from build123d import *

# Parameters (mm, degrees)
SKETCH1_R           = 2.1
BOSS_EXTRUDE1_DEPTH = 3.175
FILLET2_R           = 1
FILLET3_R           = 1


with BuildPart() as part:
    # Sketch1 → Boss-Extrude1 (new body)
    with BuildSketch(Plane.XY):
        with BuildLine():
            Line((7.553744451, 70.714270531), (-1.524, 70.714270531))
            Line((-1.524, 70.714270531), (-1.524, 132.971298819))
            Line((-1.524, 132.971298819), (-13.246972093, 161.314442451))
            Line((-13.246972093, 161.314442451), (-11.976972093, 161.314442451))
            ThreePointArc((-11.976972093, 161.314442451), (0.849692503, 157.261830841), (10.122503099, 167.006674049))
            Line((10.122503099, 167.006674049), (11.392503099, 167.006674049))
            Line((11.392503099, 167.006674049), (10.2026, 132.971298819))
            Line((10.2026, 132.971298819), (10.2026, 70.714270531))
            Line((10.2026, 70.714270531), (7.553744451, 70.714270531))
        make_face()
        with Locations((4.2926, 126.820276743)):
            Circle(SKETCH1_R, mode=Mode.SUBTRACT)
        with Locations((4.2926, 80.951718801)):
            Circle(SKETCH1_R, mode=Mode.SUBTRACT)
    extrude(amount=BOSS_EXTRUDE1_DEPTH)

    # Fillet2
    fillet2_edges = [part.edges().sort_by_distance(p)[0] for p in [
        (-11.976972093, 161.314442451, 1.5875),
        (10.122503099, 167.006674049, 1.5875),
        (10.2026, 70.714270531, 1.5875),
        (-1.524, 70.714270531, 1.5875),
        (-1.524, 132.971298819, 1.5875),
    ]]
    fillet(fillet2_edges, radius=FILLET2_R)

    # Fillet3
    # the kernel refuses this fillet: 1 mm, written as the material it takes off along each edge
    with BuildSketch(Plane(origin=(-13.246972093, 161.314442451, -3.208100544), x_dir=(1, 0, 0), z_dir=(0, 0, 1))) as fillet3_piece_1:
        with BuildLine():
            CenterArc((1.414539547, -0.803606449), FILLET3_R, 126.524113779, 75.946301344)
            Line((0.490462538, -1.185812782), (0.471980998, -1.193456909))
            Line((0.471980998, -1.193456909), (-0.01848154, -0.007644127))
            Line((-0.01848154, -0.007644127), (0, 0.02))
            ThreePointArc((0, 0.02), (0.409689249, 0.02), (0.807475277, 0.016072129))
            Line((0.807475277, 0.016072129), (0.819378498, 0))
        make_face()
    extrude(amount=9.591201087, mode=Mode.SUBTRACT)
    with BuildSketch(Plane(origin=(11.392503099, 167.006674049, -2.176149378), x_dir=(-1, 0, 0), z_dir=(0, 0, 1))) as fillet3_piece_2:
        with BuildLine():
            CenterArc((1.029802799, 0.834988847), FILLET3_R, 177.997710642, 58.616966228)
            Line((0.030413367, 0.869928276), (0.010425578, 0.870627065))
            Line((0.010425578, 0.870627065), (-0.019987789, 0.000698789))
            Line((-0.019987789, 0.000698789), (0, -0.02))
            ThreePointArc((0, -0.02), (0.239767965, -0.02), (0.468530594, -0.016699777))
            Line((0.468530594, -0.016699777), (0.479535931, 0))
        make_face()
    extrude(amount=7.527298756, mode=Mode.SUBTRACT)


solid = part.part
The listing builds one solid part. Answer for the finished solid, in the listing's coordinates (mm). A direction names the side the tool comes from. Round coordinates to 2 decimals unless told otherwise and drop trailing zeros. Write each loop counter-clockwise with the first axis right and the second up, starting at its lowest first coordinate (ties: lowest second). Pieces come first, ordered by that corner, then holes. Notation, with made-up numbers: M -32.5,31 L -17.5,31 A20 ccw -17.5,39 Z; hole C 86.25,6.5 d8. An arc over 180 degrees is marked long. Write each question's results on one line, items separated by ' | '. Start each with the question number.
(1) The part is cut by section D-D, the plane y = 107.5. Write down the section's boundary in (x, z) (3 decimals).
(2) The part is cut by section B-B, the plane z = 1.9. Write down the section's boundary in (x, y), and give its area (3 significant figures).
(3) The part is cut by section C-C, the plane x = 1.25. Write down the section's boundary in (y, z) (3 decimals), and give its area (3 significant figures).
(4) Determine the mould class of faces 1 (the flat face through (-1.524, 102, 2)), 2 (the cylindrical face through (0.51, 157.18, 1.57)), 3 (the flat face through (5, 120, 0)), 4 (the cylindrical face through (4, 128.9, 1.6)) for opening direction X: +X half, -X half, draft (parallel to the pull), parting line (faces both ways), or undercut.
(5) For faces 5 (the flat face through (4, 70.714, 2)), 6 (the flat face through (10.203, 103, 2)), determine the directions among +Z, -Z, +X, -X, +Y, -Y from which every point of the face is accessible in a straight line to the end or side of a thin tool.
(6) The part is cut by section A-A, the plane y = 159. Write down the section's boundary in (x, z) (3 decimals).
(7) Find the intervals of material crossed by line 1 (Y direction, x = 6, z = 0.2); line 2 (X direction, y = 81, z = 1.1); line 3 (X direction, y = 84, z = 0.3), in increasing order.
Worked answers:
1) outline: M -1.524,0 L 10.203,0 L 10.203,3.175 L -1.524,3.175 Z
2) outline: M -12.76,160.13 L -1.6,133.15 A1 cw -1.52,132.77 L -1.52,71.71 A1 ccw -0.52,70.71 L 9.2,70.71 A1 ccw 10.2,71.71 L 10.2,132.97 L 11.36,166.14 A1 ccw 10.91,167.01 A1 ccw 9.95,166.27 A12.7 cw -11.69,160.99 A1 ccw -12.43,161.31 A1 ccw Z; hole C 4.29,80.95 d4.2; hole C 4.29,126.82 d4.2 | area: 1,170 mm²
3) outline: M 70.714,0 L 157.372,0 L 157.372,3.175 L 70.714,3.175 Z | area: 275 mm²
4) face 1: -X half | face 2: undercut | face 3: draft | face 4: undercut
5) face 5: +Z, -Z, +X, -X, -Y | face 6: +Z, -Z, +X, -Y
6) outline: M -12.29,0 L -9.373,0 L -9.373,3.175 L -12.29,3.175 Z; M 4.737,0 L 11.113,0 L 11.113,3.175 L 4.737,3.175 Z
7) line 1: y = 70.71 to 79.73, 82.17 to 125.6, 128.04 to 159.96 | line 2: x = -1.52 to 2.19, 6.39 to 10.2 | line 3: x = -1.52 to 10.2
